Geometry check sheet. Reference: the model listing, model coordinates, mm. Face numbers are marked on the shaded views. Round coordinates to 2 decimals unless told otherwise and drop trailing zeros. Order: outer loops, then holes, each group sorted by start corner. A loop starts at its lowest first (then second) coordinate and runs counter-clockwise, first axis right, second up. Notation, with made-up numbers: (12, 72) - (21, 72) arc R16 ccw to (21, 99) - close; hole circle Ø4 at (81, 45). An arc over 180 degrees is marked (long way). Use a Markdown table: item, result. Add a question column.
(1) Gauge pin test, flat ends, axial feed: P1, Ø4, axis at x = 19, y = -12, coming from the +Z side; P2, Ø1, axis at x = 40.5, z = -56, coming from the -Y side. Record the tip position at first contact, or that the pin passes through.
(2) Section check A-A on x = 36. Record the boundary of the cut face in (y, z).
(3) Section check C-C on y = -2. Record the boundary of the cut face in (x, z).
(4) Thickness scan on line 1 along Z through (x, y) = (32, -4.75); line 2 along Y through (x, z) = (53, -16). Record the ranges inside material, lowest first. Write a range as [from, to].
(5) Section check B-B on z = -71. Record the boundary of the cut face in (x, y), then the cut area to 3 significant figures.
(6) Mould release check, pull along Y, two halves, no side actions. Record for the marked faces 1, 2 and 3: released by +Y, released by -Y, zero draft, split by the parting line, or undercut.
Autodesk Inventor part; units mm, degrees
ref_plane "Work Plane1" through (54, 0, -84) normal (0, 0, -1) x (-1, 0, 0)
ref_plane "YZ Plane" through (0, 0, 0) normal (1, 0, 0) x (0, 1, 0)
ref_plane "XZ Plane" through (0, 0, 0) normal (0, 1, 0) x (-1, 0, 0)
sketch "Sketch1" plane through (0, 0, 0) normal (0, 1, 0) x (-1, 0, 0)
  line L0 (0, 0) -> (-56, 0)
  line L1 (-56, 0) -> (-56, -84)
  line L2 (-56, -84) -> (0, -84)
  line L3 (0, -84) -> (0, 0)
  point P0 (-28, -84)
  dimension "d0" = 56
  dimension "d1" = 84
extrude "Extrusion1" add sketch "Sketch1" along normal blind 1
fillet "Fillet1" radius 2 1 edges at (0, 0.5, 0)
fillet "Fillet2" radius 2 1 edges at (56, 0.5, 0)
fillet "Fillet3" radius 2 1 edges at (56, 0.5, -84)
fillet "Fillet4" radius 2 1 edges at (0, 0.5, -84)
sketch "Sketch2" plane through (0, 1, 0) normal (0, 1, 0) x (1, 0, 0)
  point P0 (0, 0)
ref_plane "Work Plane1" through (54, 0, -84) normal (0, 0, -1) x (-1, 0, 0)
sketch "Sketch3" plane through (54, 0, -84) normal (0, 0, -1) x (-1, 0, 0)
  line L0 (-2, 1) -> (0, 1)
  line L1 (-2, 1) -> (54, 1)
  line L2 (54, 1) -> (54, -14)
  line L3 (54, -14) -> (-2, -14)
  line L4 (-2, -14) -> (-2, 1)
  point P0 (54, 0)
  dimension "d9" = 0
  dimension "d10" = 15
extrude "Extrusion2" add sketch "Sketch3" along normal blind 1
properties part number "cover"
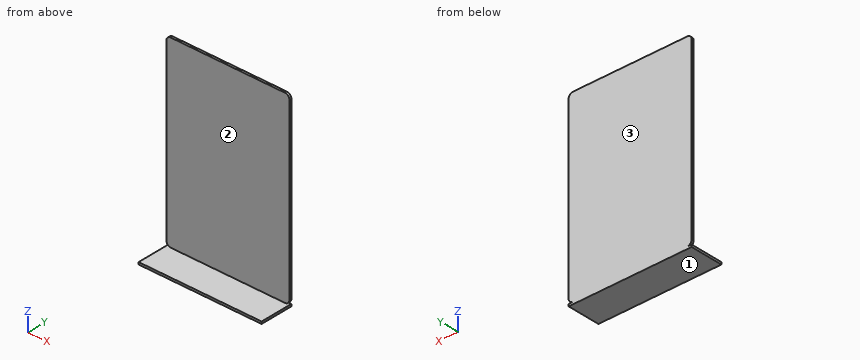
Check sheet entries:
| question | item | result |
|---|---|---|
| 1 | P1 | stops at z = -84 |
| 1 | P2 | stops at y = 0 |
| 2 | outline | (-14, -85) - (1, -85) - (1, 0) - (0, 0) - (0, -84) - (-14, -84) - close |
| 3 | outline | (0, -85) - (56, -85) - (56, -84) - (0, -84) - close |
| 4 | line 1 | z = [-85, -84] |
| 4 | line 2 | y = [0, 1] |
| 5 | outline | (0, 0) - (56, 0) - (56, 1) - (0, 1) - close |
| 5 | area | 56.0 mm2 |
| 6 | face 1 | zero draft |
| 6 | face 2 | released by -Y |
| 6 | face 3 | released by +Y |
